```python
from build123d import *

# Parameters (mm, degrees)
F3_W     = 72
F3_H     = 72
F3_R     = 1.2
F3_R_2   = 35
F4_DEPTH = 3


with BuildPart() as f1:
    # F0 (on Right) → F1 (revolve)
    with BuildSketch(Plane.YZ):
        Polygon((2, 35), (-3, 35), (-3, 34), (1, 31), (2, 31), align=None)
    revolve(axis=Axis((0, 1.602868, 0), (0, -1, 0)))

    # F3 (on offset) → F4 (join)
    with BuildSketch(Plane.XZ.offset(1)):
        Rectangle(F3_W, F3_H)
        with Locations((-28, -28)):
            Circle(F3_R, mode=Mode.SUBTRACT)
        with Locations((28, -28)):
            Circle(F3_R, mode=Mode.SUBTRACT)
        with Locations((-28, 28)):
            Circle(F3_R, mode=Mode.SUBTRACT)
        Circle(F3_R_2, mode=Mode.SUBTRACT)
        with Locations((28, 28)):
            Circle(F3_R, mode=Mode.SUBTRACT)
    extrude(amount=-F4_DEPTH)


solid = f1.part
```
The model under review builds one solid part; all positions refer to its coordinate system, in mm. A direction names the side the tool comes from. Round coordinates to 2 decimals unless told otherwise and drop trailing zeros. Write each loop counter-clockwise with the first axis right and the second up, starting at its lowest first coordinate (ties: lowest second). Pieces come first, ordered by that corner, then holes.
(1) Wall thickness on L1, parallel to Z at x = -28, y = 0; L2, parallel to X at y = -2.2, z = -1.5; L3, parallel to Y at x = 28.5, z = 20.5: over which ranges is each line inside the solid? List them lowest first.
(2) Mouldability with a two-part tool opening along X and no side actions: class faces 3 (the flat face through (-36, 0, -1)), 4 (the cylindrical face through (28.554, 0.479, -29.065)), 5 (the flat face through (-19, -1, 30)) as +X half, -X half, draft (parallel to the pull), parting line (faces both ways), or undercut.
(3) We need section B-B on x = 0. Give the boundary of the cut face in (y, z), and give its area (3 significant figures).
(4) We need section C-C on y = 0.25. Give the boundary of the cut face in (x, z) (1 decimal), and give its area (3 significant figures).
(5) Machinability: for faces 1 (the cylindrical face through (-10.513, -2.014, 33.384)), 2 (the cylindrical face through (-27.446, 0.479, 26.935)), which of the approach directions +Z, -Z, +X, -X, +Y, -Y give a long, thin tool a straight path to every point of the face, cutting with its end or side? Answer none if there is none.
(6) We need section A-A on z = 0. Give the boundary of the cut face in (x, y), and give its area (3 significant figures).
(7) Insertion check: pin 1 (3 mm diameter, centred on x = 26.5, z = 25, fed in from -Y); pin 2 (10 mm diameter, centred on x = 12.5, z = -24.5, fed in from -Y). Each pin has a flat end and moves straight along its axis. Give the tip position at first contact, or say it passes through.
(8) We need section D-D on x = 28. Give the number of separate pieces and of enclosed holes in the cut face, and give its area (3 significant figures).
Findings below:
1. L1: z = -36 to -29.2, -26.8 to -14.97, 14.97 to 26.8, 29.2 to 36
1. L2: x = -34.97 to -33.37, 33.37 to 34.97
1. L3: y = -1 to 2
2. face 3: -X half
2. face 4: undercut
2. face 5: draft
3. outline: (-3, -35) - (-1, -35) - (-1, -36) - (2, -36) - (2, -31) - (1, -31) - (-3, -34) - close; (-3, 34) - (1, 31) - (2, 31) - (2, 36) - (-1, 36) - (-1, 35) - (-3, 35) - close
3. area: 34.0 mm2
4. outline: (-36, -36) - (36, -36) - (36, 36) - (-36, 36) - close; hole circle Ø63.1 at (0, 0); hole circle Ø2.4 at (-28, -28); hole circle Ø2.4 at (-28, 28); hole circle Ø2.4 at (28, -28); hole circle Ø2.4 at (28, 28)
4. area: 2,040 mm2
5. face 1: -Y
5. face 2: +Y, -Y
6. outline: (-36, -1) - (-35, -1) - (-35, -3) - (-34, -3) - (-31, 1) - (-31, 2) - (-36, 2) - close; (31, 1) - (34, -3) - (35, -3) - (35, -1) - (36, -1) - (36, 2) - (31, 2) - close
6. area: 34.0 mm2
7. pin 1: stops at y = -3
7. pin 2: stops at y = -1.01
8. separate pieces: 4
8. enclosed holes: 0
8. area: 128 mm2
